Autodesk Fusion 360 part; units mm, degrees
sketch "Sketch1" plane through (0, 0, 0) normal (0, 1, 0) x (1, 0, 0)
  circle A0 centre (0, 0) radius 1.2
  circle A1 centre (0, 0) radius 2.4
  dimension "d1" = 2.4
  dimension "d2" = 1.2
extrude "Extrude1" add sketch "Sketch1" along normal blind 13.5
sketch "Sketch2" plane through (0, 13.5, 0) normal (0, 1, 0) x (-1, 0, 0)
  circle A0 centre (0, 0) radius 1.2
  circle A1 centre (0, 0) radius 2.4
  circle A2 centre (0, 0) radius 1.2
  circle A3 centre (0, 0) radius 2.4
extrude "Extrude2" add sketch "Sketch2" along normal blind 1.2 contours A0 A2 | A1 A3
sketch "Sketch3" plane through (0, 14.7, 0) normal (0, 1, 0) x (-1, 0, 0)
  circle A0 centre (0, 0) radius 2.4
  circle A1 centre (0, 0) radius 3.5
  dimension "d11" = 7
extrude "Extrude3" add sketch "Sketch3" along normal blind 14 contours A0 | A1
extrude "Extrude4" add 1 faces at (0.7915, 28.7, 0.6312) along direction (0, 1, 0) blind 7 draft -22.5
fillet "Fillet1" radius 0.8 1 faces at (-0.4122, 35.7, -0.15)
fillet "Fillet2" radius 2.5 1 edges at (3.2631, 28.7, -1.2657)
sketch "Sketch4" plane through (0, 14.7, 0) normal (0, -1, 0) x (1, 0, 0)
  circle A0 centre (0, 0) radius 3.5
  circle A1 centre (0, 0) radius 2.4
sketch "Sketch5" plane through (0, 0, 0) normal (0, 1, 0) x (1, 0, 0)
  circle A0 centre (0, 0) radius 3.5
  circle A1 centre (0, 0) radius 3.3
  dimension "d20" = 7
  dimension "d21" = 6.6
extrude "Extrude7" cut sketch "Sketch5" along normal blind 20.8 and the other way blind -21.2
extrude "Extrude8" cut sketch "Sketch5" along normal blind 21.6 and the other way blind -22
extrude "Extrude9" cut sketch "Sketch5" along normal blind 22.4 and the other way blind -22.8
extrude "Extrude10" cut sketch "Sketch5" along normal blind 23.2 and the other way blind -23.6
extrude "Extrude11" cut sketch "Sketch5" along normal blind 24 and the other way blind -24.4
extrude "Extrude12" cut sketch "Sketch5" along normal blind 24.8 and the other way blind -25.2
extrude "Extrude13" cut sketch "Sketch5" along normal blind 25.6 and the other way blind -26
extrude "Extrude15" cut sketch "Sketch1" along normal blind 32.4 contours A0
equation "d1 = ProbeDiameter + ProbeDeiameterClearence"
equation "d2 = WallThickness"
equation "d3 = ProbeLenght"
equation "d5 = WallThickness"
equation "ProbeDiameter = 2.4 mm"
equation "ProbeDeiameterClearence = 0 mm"
equation "ProbeLenght = 13.5 mm"
equation "WallThickness = 1.2 mm"
equation "RidgeBaseDist = 19.6 mm"
equation "RidgeDistIncrement = 0.4 mm"
equation "RidgeSecondDist = -19.2 mm"
equation "RidgeCutGap = -0.4 mm"
equation "d34 = RidgeBaseDist + ( 3 * RidgeDistIncrement )"
equation "d36 = RidgeSecondDist + ( 5 * RidgeCutGap )"
equation "d38 = RidgeBaseDist + ( 5 * RidgeDistIncrement )"
equation "d40 = RidgeSecondDist + ( 7 * RidgeCutGap )"
equation "d42 = RidgeBaseDist + ( 7 * RidgeDistIncrement )"
equation "d44 = RidgeSecondDist + ( 9 * RidgeCutGap )"
equation "d46 = RidgeBaseDist + ( 9 * RidgeDistIncrement )"
equation "d48 = RidgeSecondDist + ( 11 * RidgeCutGap )"
equation "d50 = RidgeBaseDist + ( 11 * RidgeDistIncrement )"
equation "d52 = RidgeSecondDist + ( 13 * RidgeCutGap )"
equation "d54 = RidgeBaseDist + ( 13 * RidgeDistIncrement )"
equation "d56 = RidgeSecondDist + ( 15 * RidgeCutGap )"
equation "d58 = RidgeBaseDist + ( 15 * RidgeDistIncrement )"
equation "d60 = RidgeSecondDist + ( 17 * RidgeCutGap )"
Build history of the part. All positions in model axes, mm. A direction names the side the tool comes from. Round coordinates to 2 decimals unless told otherwise and drop trailing zeros. Loops run counter-clockwise (first coordinate to the right, second up) from the corner with the lowest first, then second, coordinate; pieces in that order, holes last. Notation, with made-up numbers: M 40,-25 L 67,-25 A21 ccw 67,-10 Z; hole C 66,-24.5 d4. An arc over 180 degrees is marked long. Answer as CSV lines item,"result".
1. 3-axis set-ups, long thin cutter, end or side, ignore diameter. For faces 4 (the cylindrical face through (-2.43, 21, -2.23)), 5 (the cylindrical face through (-3.233, 22.997, 1.341)): which of +Z, -Z, +X, -X, +Y, -Y reach the whole face in a straight line?
Resolved:
face 4,"none"
face 5,"+Y, -Y"
2. Flat gauge pins, fed straight in: P1, Ø3, axis at y = 8, z = 1, coming from the +X side; P2, Ø2, axis at y = 30.5, z = -1, coming from the +X side; P3, Ø1.5, axis at x = 0, z = 0, coming from the -Y side. Where does each tip first touch, or does it go through?
Resolved:
P1,"stops at x = 2.4"
P2,"stops at x = 3.08"
P3,"stops at y = 32.4"
3. Cut at A-A on y = 12. Write the cut outline in (x, z).
Resolved:
outline,"C 0,0 d4.8; hole C 0,0 d2.4"
4. Wall check: probe 1 along X at (y, z) = (2, 0); probe 2 along Z at (x, y) = (0, 19); probe 3 along Z at (x, y) = (0, 21). Give the ranges that are in metal, low to high. Write a range as [from, to].
Resolved:
probe 1,"x = [-2.4, -1.2], [1.2, 2.4]"
probe 2,"z = [-3.5, -1.2], [1.2, 3.5]"
probe 3,"z = [-3.3, -1.2], [1.2, 3.3]"
5. Two-plate mould, pull along Y, no slides. Class faces 1 (the cylindrical face through (-3.233, 22.197, 1.341)), 2 (the cylindrical face through (-2.43, 25, -2.23)), 3 (the flat face through (0, 32.4, 0)): released by +Y, released by -Y, zero draft, split by the parting line, or undercut.
Resolved:
face 1,"zero draft"
face 2,"undercut"
face 3,"released by -Y"
